Here's the drawing with two shaded views (mm, measured from the low corner). I have some questions. Give positions to 0.01 mm unless a question says otherwise; leave off trailing zeros. Write each loop counter-clockwise with the first axis right and the second up, starting at its lowest first coordinate (ties: lowest second). Pieces come first, ordered by that corner, then holes. Notation, with made-up numbers: (-2.75, -28) -> (55.25, -28) arc R34 cw to (55.25, 4) -> close; hole circle Ø11 at (6.5, 32). An arc over 180 degrees is marked (long way). One line per item, written item: value.
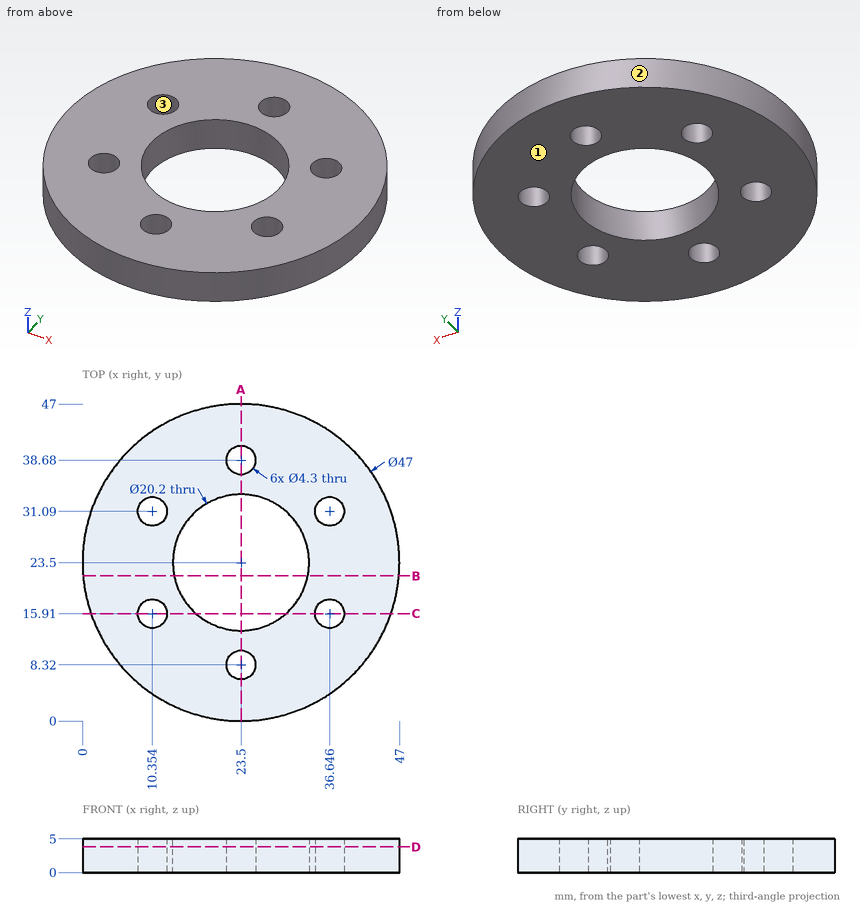
1) If we section it at B-B (y = 21.5): Write out the boundary of the cut face in (x, z) (1 decimal).
Answer list:
outline: (0.1, 0) -> (13.6, 0) -> (13.6, 5) -> (0.1, 5) -> close; (33.4, 0) -> (46.9, 0) -> (46.9, 5) -> (33.4, 5) -> close
2) Will these pins go through, and if not, where does the flat tip stop? pin 1 (1.5 mm diameter, centred on x = 41.5, z = 2.5, fed in from +Y); pin 2 (3 mm diameter, centred on x = 21, z = 2, fed in from -Y).
Answer list:
pin 1: stops at y = 39.46
pin 2: stops at y = 0.02
3) If we section it at A-A (x = 23.5): Write out the boundary of the cut face in (y, z), and give its area (3 significant figures).
Answer list:
outline: (0, 0) -> (6.17, 0) -> (6.17, 5) -> (0, 5) -> close; (10.47, 0) -> (13.4, 0) -> (13.4, 5) -> (10.47, 5) -> close; (33.6, 0) -> (36.53, 0) -> (36.53, 5) -> (33.6, 5) -> close; (40.83, 0) -> (47, 0) -> (47, 5) -> (40.83, 5) -> close
area: 91.0 mm^2
4) I need wall thicknesses on L1, parallel to X at y = 32, z = 4.4 (1 decimal); L2, parallel to Y at x = 23.5, z = 2.65; L3, parallel to X at y = 15.91, z = 1.15 (1 decimal). Which ranges of each line are inside material? Lowest first, please.
Answer list:
L1: x = 1.6 to 8.4, 12.3 to 18, 29 to 34.7, 38.6 to 45.4
L2: y = 0 to 6.17, 10.47 to 13.4, 33.6 to 36.53, 40.83 to 47
L3: x = 1.3 to 8.2, 12.5 to 16.8, 30.2 to 34.5, 38.8 to 45.7
5) If we section it at D-D (z = 3.85): Write out the boundary of the cut face in (x, y), and give its area (3 significant figures).
Answer list:
outline: circle Ø47 at (23.5, 23.5); hole circle Ø4.3 at (10.35, 15.91); hole circle Ø4.3 at (10.35, 31.09); hole circle Ø20.2 at (23.5, 23.5); hole circle Ø4.3 at (23.5, 8.32); hole circle Ø4.3 at (23.5, 38.68); hole circle Ø4.3 at (36.65, 15.91); hole circle Ø4.3 at (36.65, 31.09)
area: 1,330 mm^2
6) If we section it at C-C (y = 15.91): Write out the boundary of the cut face in (x, z), and give its area (3 significant figures).
Answer list:
outline: (1.26, 0) -> (8.2, 0) -> (8.2, 5) -> (1.26, 5) -> close; (12.5, 0) -> (16.84, 0) -> (16.84, 5) -> (12.5, 5) -> close; (30.16, 0) -> (34.5, 0) -> (34.5, 5) -> (30.16, 5) -> close; (38.8, 0) -> (45.74, 0) -> (45.74, 5) -> (38.8, 5) -> close
area: 113 mm^2
7) We'd pull the mould along Y, two halves only. Please class the marked faces 1, 2 and 3: released by +Y, released by -Y, zero draft, split by the parting line, or undercut.
Answer list:
face 1: zero draft
face 2: split by the parting line
face 3: undercut
